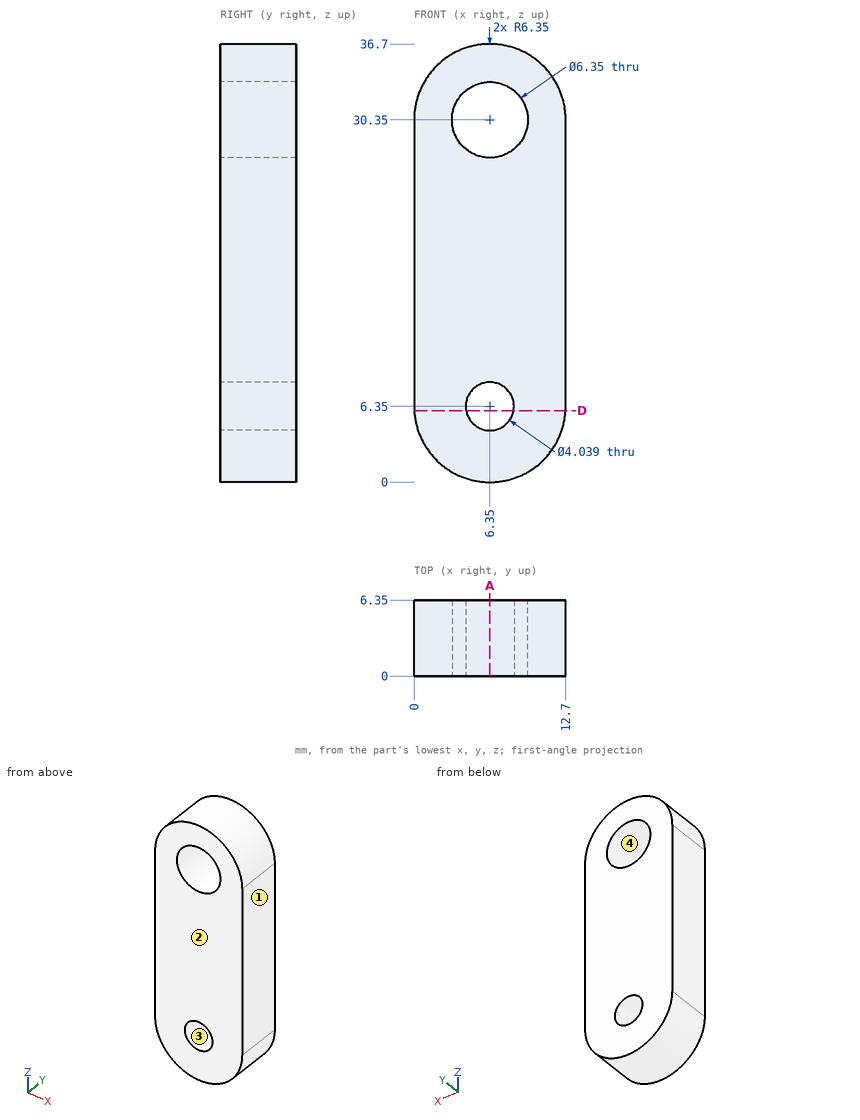
Can you work these out from the drawing? Everything is in mm from the part's minimum corner. Give positions to 0.01 mm unless a question says otherwise; leave off trailing zeros. Order: outer loops, then holes, each group sorted by start corner. A loop starts at its lowest first (then second) coordinate and runs counter-clockwise, first axis right, second up.
Item 1: If we section it at A-A, the plane x = 6.35: Count the separate pieces of the cut face and the enclosed holes in it, plus the area to 3 significant figures.
Item 2: If we mould it in two halves opening along X, with no side actions, what happens to the marked faces 1, 2, 3 and 4? For each: pulls with the +X half, pulls with the -X half, needs draft (parallel to the pull), parting line crosses it, or undercut.
Item 3: If we section it at D-D, the plane z = 6: Write out the boundary of the cut face in (x, y).
Item 4: I need wall thicknesses on line 1 (Z direction, x = 6.35, y = 4) (1 decimal); line 2 (X direction, y = 3.75, z = 30.35) (1 decimal); line 3 (Z direction, x = 8, y = 6) (1 decimal). Which ranges of each line are inside material? Lowest first, please.
Item 5: I'm going to push a flat-ended pin straight in: pin 1 (4.5 mm diameter, centred on x = 6.35, z = 6.35, fed in from -Y). Where does the tip first touch, or does it pass through?
Values:
1. separate pieces: 3
1. enclosed holes: 0
1. area: 167 mm2
2. face 1: pulls with the +X half
2. face 2: needs draft
2. face 3: undercut
2. face 4: undercut
3. outline: (0.01, 0) - (4.36, 0) - (4.36, 6.35) - (0.01, 6.35) - close; (8.34, 0) - (12.69, 0) - (12.69, 6.35) - (8.34, 6.35) - close
4. line 1: z = 0 to 4.3, 8.4 to 27.2, 33.5 to 36.7
4. line 2: x = 0 to 3.2, 9.5 to 12.7
4. line 3: z = 0.2 to 5.2, 7.5 to 27.6, 33.1 to 36.5
5. pin 1: stops at y = 0
